Could you check a few things on this model? Use its own coordinates, in mm. A direction names the side the tool comes from. Give positions to 0.01 mm unless a question says otherwise; leave off trailing zeros. Write each loop counter-clockwise with the first axis right and the second up, starting at its lowest first coordinate (ties: lowest second). Pieces come first, ordered by that corner, then holes. Notation, with made-up numbers: (-10, -14.75) - (18, -14.75) arc R31 ccw to (18, 17.25) - close; hole circle Ø8 at (11.25, 7). An arc over 180 degrees is marked (long way). Write item = value, one per line.
from build123d import *

# Parameters (mm, degrees)
F0_R     = 35
F1_DEPTH = 400
F2_R     = 5
F3_DEPTH = 30
F4_DEPTH = 430
F6_DEPTH = 30
F7_DEPTH = 430


with BuildPart() as f1:
    # F0 (on Front) → F1 (new body)
    with BuildSketch(Plane.XZ):
        Circle(F0_R)
    extrude(amount=F1_DEPTH)

    # F2 (on Front) → F3 (join)
    with BuildSketch(Plane.XZ):
        Circle(F2_R)
    extrude(amount=-F3_DEPTH)

    # F2 (on Front) → F4 (join)
    with BuildSketch(Plane.XZ):
        Circle(F2_R)
    extrude(amount=F4_DEPTH)

    # F5 (on face) → F6 (join, symmetric)
    with BuildSketch(Plane.XZ.offset(400)):
        with BuildLine():
            ThreePointArc((2.5, -4.3301270189), (0, -5), (-2.5, -4.3301270189))
            Line((-2.5, -4.3301270189), (-2.5, -10))
            Line((-2.5, -10), (2.5, -10))
            Line((2.5, -10), (2.5, -4.3301270189))
        make_face()
    extrude(amount=F6_DEPTH, both=True)

    # F5 (on face) → F7 (join)
    with BuildSketch(Plane.XZ.offset(400)):
        with BuildLine():
            ThreePointArc((2.5, -4.3301270189), (0, -5), (-2.5, -4.3301270189))
            Line((-2.5, -4.3301270189), (-2.5, -10))
            Line((-2.5, -10), (2.5, -10))
            Line((2.5, -10), (2.5, -4.3301270189))
        make_face()
    extrude(amount=-F7_DEPTH)


solid = f1.part
1. If we section it at B-B, the plane y = -54: Please give me the cut outline in (x, z), and give its area (3 significant figures).
Filled sheet:
outline = circle Ø70 at (0, 0)
area = 3,850 mm2
2. If we section it at C-C, the plane x = -16: Please give me the cut outline in (y, z), and give its area (3 significant figures).
Filled sheet:
outline = (-400, -31.13) - (0, -31.13) - (0, 31.13) - (-400, 31.13) - close
area = 24,900 mm2
3. Which directions (+Z, -Z, +X, -X, +Y, -Y) give clear straight access to the entire face, cutting with the end or side of a thin tool? Please do faces 1 (the face through (0, 30, -2)), 2 (the face through (0, -415, 5)), 3 (the face through (0, 15, 5)).
Filled sheet:
face_1 = +Z, -Z, +X, -X, +Y
face_2 = -Y
face_3 = +Y
4. For pin 1 (6 mm diameter, centred on x = -18.5, z = -20.5, fed in from -Y); pin 2 (5 mm diameter, centred on y = -358, z = -4, fed in from +X); pin 3 (2 mm diameter, centred on y = -29, z = -15, fed in from +X); pin 4 (10 mm diameter, centred on y = -60, z = -3, fed in from -X), each with a flat end and sliding along its axis, tell me the tip position at first contact or that it passes through.
Filled sheet:
pin_1 = -400
pin_2 = 34.97
pin_3 = 32.08
pin_4 = -35
5. If we section it at D-D, the plane z = 26.5: Please give me the cut outline in (x, y).
Filled sheet:
outline = (-22.86, -400) - (22.86, -400) - (22.86, 0) - (-22.86, 0) - close
6. If we section it at A-A, the plane z = 0: Please give me the cut outline in (x, y).
Filled sheet:
outline = (-35, -400) - (-5, -400) - (-5, -430) - (5, -430) - (5, -400) - (35, -400) - (35, 0) - (5, 0) - (5, 30) - (-5, 30) - (-5, 0) - (-35, 0) - close
7. I need wall thicknesses on line 1 (Y direction, x = -11, z = -14); line 2 (X direction, y = -227, z = 1); line 3 (Z direction, x = 20.5, y = -79.5). Which ranges of each line are inside material? Lowest first, please.
Filled sheet:
line_1 = -400 to 0
line_2 = -34.99 to 34.99
line_3 = -28.37 to 28.37
